The listing builds one solid part. Answer for the finished solid, in the listing's coordinates (mm). A direction names the side the tool comes from. Coordinates: 2 decimals unless noted, no trailing zeros. Order: outer loops, then holes, each group sorted by start corner. A loop starts at its lowest first (then second) coordinate and runs counter-clockwise, first axis right, second up. Notation, with made-up numbers: (57.5, 52.25) -> (98.5, 52.25) arc R38 ccw to (98.5, 90.25) -> close; hole circle Ø11 at (32, -19). An arc over 180 degrees is marked (long way). Answer in a Markdown table with one row per item. Add a question column.
```python
from build123d import *

# Parameters (mm, degrees)
PAD017_DEPTH           = 5
PAD020_DEPTH           = 6.25
SKETCH118_W            = 5.2
SKETCH118_H            = 1.65
PAD087_DEPTH           = 7.5
SKETCH116_W            = 5.2
SKETCH116_H            = 1.65
PAD088_DEPTH           = 5
SKETCH117_W            = 5.2
SKETCH117_H            = 1.65
PAD089_DEPTH           = 7.5
LINEARPATTERN028_COUNT = 2
LINEARPATTERN028_PITCH = 3.3


with BuildPart() as obj1:
    # Sketch034 → Pad017 (new body)
    with BuildSketch(Plane.XY):
        with BuildLine():
            Line((-1.35, -1.8), (-1.35, 6))
            ThreePointArc((0, 7.35), (-0.954594, 6.954594), (-1.35, 6))
            Line((0, 9), (0, 7.35))
            Line((-2.6, 9), (0, 9))
            Line((-2.6, -1.8), (-2.6, 9))
            Line((-3.85, -1.8), (-2.6, -1.8))
            ThreePointArc((-3.85, -1.8), (-3.439949, -2.789949), (-2.45, -3.2))
            Line((-1.35, -3.2), (-2.45, -3.2))
            Line((-1.35, -1.8), (-1.35, -3.2))
        make_face()
    extrude(amount=PAD017_DEPTH)

    # Sketch037 → Pad020 (join)
    with BuildSketch(Plane.XY):
        Polygon((-1.35, 0.2), (-1.35, 1.6), (-2.6, 1.6), (-3.85, 1.6), (-3, 0.2), (-2.6, 0.2), align=None)
    extrude(amount=PAD020_DEPTH)


with BuildPart() as obj2:
    # Mirror001: instance of _obj1
    add(obj1.part.mirror(Plane(origin=(0, 0, 0), x_dir=(0, 1, 0), z_dir=(-1, 0, 0))))


with BuildPart() as body044:
    # Fusion001 base: copy of _obj1
    add(obj1.part)

    # Fusion001: union _obj2)
    add(obj2.part)

    # Sketch118 → Pad087 (new body)
    with BuildSketch(Plane.XY):
        with Locations((0, 8.175)):
            Rectangle(SKETCH118_W, SKETCH118_H)
    extrude(amount=PAD087_DEPTH)

    # Sketch116 → Pad088 (join)
    with BuildSketch(Plane.XY):
        with Locations((0, 9.825)):
            Rectangle(SKETCH116_W, SKETCH116_H)
    pad088 = extrude(amount=PAD088_DEPTH)

    # Sketch117 → Pad089 (join)
    with BuildSketch(Plane.XY):
        with Locations((0, 11.475)):
            Rectangle(SKETCH117_W, SKETCH117_H)
    pad089 = extrude(amount=PAD089_DEPTH)

    # LinearPattern028: Pad089, Pad088 ×2
    with Locations(*[(0, i * LINEARPATTERN028_PITCH, 0) for i in range(1, LINEARPATTERN028_COUNT)]):
        add(pad089)
        add(pad088)


solid = body044.part
```
Q1. For faces 1 (the face through (2.6, 9, 3)), 2 (the face through (2, 1, 6.25)), 3 (the face through (-3, -1.8, 2)), 4 (the face through (0, 13, 5)), determine the directions among +Z, -Z, +X, -X, +Y, -Y from which every point of the face is accessible in a straight line to the end or side of a thin tool.
Q2. A cutting plane is placed at D-D (z = 1.75). Determine the outline of the cut face in (x, y).
Q3. Given pin 1 (1.5 mm diameter, centred on x = 2.5, y = 8.5, fed in from -Z); pin 2 (2 mm diameter, centred on x = 1, z = 6, fed in from -Y); pin 3 (0.6 mm diameter, centred on y = -1, z = 1.5, fed in from -X); pin 4 (3 mm diameter, centred on x = -2, y = -2, fed in from +Z), each flat-ended and moving along its own axis, determine where each tip first touches the part or whether it passes through.
Q4. A cutting plane is placed at B-B (y = -1). Determine the outline of the cut face in (x, z).
Q5. A cutting plane is placed at C-C (x = 3.25). Determine the outline of the cut face in (y, z).
Q6. Straight lines are drawn through the part: line 1 (Y direction, x = 2, z = 6); line 2 (X direction, y = 4.25, z = 3.5); line 3 (X direction, y = 13.25, z = 2). For each, find the intervals that lie inside material, in ascending order.
Q7. Determine the mould class of faces 5 (the face through (0, 10, 5)), 6 (the face through (-2.6, -1, 2)), 7 (the face through (-1.35, 1, 2)) for opening direction X: +X half, -X half, draft (parallel to the pull), parting line (faces both ways), or undercut.
Q8. A cutting plane is placed at A-A (z = 5.5). Determine the outline of the cut face in (x, y), then the cut area to 4 significant figures.
Returned:
| question | item | result |
|---|---|---|
| 1 | face 1 | +Z, -Z, +X, +Y |
| 1 | face 2 | +Z, +X, -X, -Y |
| 1 | face 3 | +Z, -Z, -X |
| 1 | face 4 | +Z, +X, -X |
| 2 | outline | (-3.85, -1.8) arc R1.4 ccw to (-2.45, -3.2) -> (-1.35, -3.2) -> (-1.35, 6) arc R1.35 cw to (0, 7.35) arc R1.35 cw to (1.35, 6) -> (1.35, -3.2) -> (2.45, -3.2) arc R1.4 ccw to (3.85, -1.8) -> (2.6, -1.8) -> (2.6, 0.2) -> (3, 0.2) -> (3.85, 1.6) -> (2.6, 1.6) -> (2.6, 15.6) -> (-2.6, 15.6) -> (-2.6, 1.6) -> (-3.85, 1.6) -> (-3, 0.2) -> (-2.6, 0.2) -> (-2.6, -1.8) -> close |
| 3 | pin 1 | stops at z = 0 |
| 3 | pin 2 | stops at y = 0.2 |
| 3 | pin 3 | stops at x = -2.6 |
| 3 | pin 4 | stops at z = 5 |
| 4 | outline | (-2.6, 0) -> (-1.35, 0) -> (-1.35, 5) -> (-2.6, 5) -> close; (1.35, 0) -> (2.6, 0) -> (2.6, 5) -> (1.35, 5) -> close |
| 5 | outline | (-2.95, 0) -> (-1.8, 0) -> (-1.8, 5) -> (-2.95, 5) -> close; (0.61, 0) -> (1.6, 0) -> (1.6, 6.25) -> (0.61, 6.25) -> close |
| 6 | line 1 | y = 0.2 to 1.6, 7.35 to 9, 10.65 to 12.3, 13.95 to 15.6 |
| 6 | line 2 | x = -2.6 to -1.35, 1.35 to 2.6 |
| 6 | line 3 | x = -2.6 to 2.6 |
| 7 | face 5 | draft |
| 7 | face 6 | -X half |
| 7 | face 7 | undercut |
| 8 | outline | (-3.85, 1.6) -> (-3, 0.2) -> (-1.35, 0.2) -> (-1.35, 1.6) -> close; (-2.6, 7.35) -> (2.6, 7.35) -> (2.6, 9) -> (-2.6, 9) -> close; (-2.6, 10.65) -> (2.6, 10.65) -> (2.6, 12.3) -> (-2.6, 12.3) -> close; (-2.6, 13.95) -> (2.6, 13.95) -> (2.6, 15.6) -> (-2.6, 15.6) -> close; (1.35, 0.2) -> (3, 0.2) -> (3.85, 1.6) -> (1.35, 1.6) -> close |
| 8 | area | 31.55 mm² |
